Work out the finished part from the listing and answer in its coordinate system (mm). A direction names the side the tool comes from. Coordinates: 2 decimals unless noted, no trailing zeros. Order: outer loops, then holes, each group sorted by start corner. A loop starts at its lowest first (then second) coordinate and runs counter-clockwise, first axis right, second up. Notation, with made-up numbers: (-34, 75.25) -> (-24, 75.25) arc R10 ccw to (-24, 91.25) -> close; hole circle Ø10 at (63.25, -24.75). An arc over 180 degrees is marked (long way). Write item = value, one per line. Start each with the question number.
Q1. The part is cut by section D-D, the plane z = -15. Determine the outline of the cut face in (x, y), plus the area to 3 significant figures.
Q2. Straight lines are drawn through the part: L1, parallel to X at y = -9.75, z = -32.5; L2, parallel to X at y = 1, z = 28.5; L3, parallel to Y at x = 25, z = -16.5. For each, find the intervals that lie inside material, in ascending order. Write a range as from..to.
Q3. Which of the six approach directions +Z, -Z, +X, -X, +Y, -Y give full straight-line access (tool end or side, diameter ignored) to faces 4 (the flat face through (4, -5, 22)), 5 (the cylindrical face through (35.593, -7.168, -40.672)), 6 (the cylindrical face through (4.6, -0.1, 21.8))?
Q4. For a pull along Z with two mould halves and no side action, classify faces 1 (the cylindrical face through (34.73, -7.17, 41.3)), 2 (the flat face through (0, 2, 0)), 3 (the cylindrical face through (15.04, 2.46, -32.63)) as +Z half, -Z half, draft (parallel to the pull), parting line (faces both ways), or undercut.
Q5. Flat-ended cylindrical pins translate along their axes: pin 1 (10 mm diameter, centred on x = 19, y = -16, fed in from -Z); pin 2 (10.5 mm diameter, centred on x = 7, z = 25, fed in from +Y); pin 3 (1.5 mm diameter, centred on x = 33.5, y = 2, fed in from -Z); pin 4 (12 mm diameter, centred on x = 29, z = 32.5, fed in from +Y). Find the tip coordinate at first contact, or state that the pin passes through.
Q6. The part is cut by section A-A, the plane y = -14. Determine the outline of the cut face in (x, z).
Q7. The part is cut by section C-C, the plane x = 29. Determine the outline of the cut face in (y, z), plus the area to 3 significant figures.
Q8. The part is cut by section B-B, the plane x = 7. Determine the outline of the cut face in (y, z).
```python
from build123d import *
from build123d.topology import SkipClean

# Parameters (mm, degrees)
SKETCH1_R                = 4
SKETCH1_R_2              = 7.5
BOSS_EXTRUDE1_DEPTH      = 5
BOSS_EXTRUDE2_START      = -5
SKETCH1_3_R              = 7
SKETCH1_3_R_2            = 4
BOSS_EXTRUDE2_DEPTH      = 5
BOSS_EXTRUDE3_DEPTH      = 5
BOSS_EXTRUDE3_DEPTH_BACK = 19
SKETCH1_4_R              = 10.5
SKETCH1_4_R_2            = 7.5


with BuildPart() as part:
    # Sketch1 → Boss-Extrude1 (new body)
    with BuildSketch(Plane(origin=(0, 0, 0), x_dir=(1, 0, 0), z_dir=(0, 1, 0))):
        with BuildLine():
            Line((2, -30), (2.101020514, -30))
            ThreePointArc((2.101020514, -30), (5.066288205, -31.727611663), (8.496335544, -31.838200051))
            ThreePointArc((8.496335544, -31.838200051), (14.961261821, -32.591823522), (19.59300275, -37.164590308))
            ThreePointArc((19.59300275, -37.164590308), (35.168768008, -40.996840663), (36.348469228, -25))
            ThreePointArc((36.348469228, -25), (25.843366656, 0), (36.348469228, 25))
            ThreePointArc((36.348469228, 25), (35.168768008, 40.996840663), (19.59300275, 37.164590308))
            ThreePointArc((19.59300275, 37.164590308), (14.961261821, 32.591823522), (8.496335544, 31.838200051))
            ThreePointArc((8.496335544, 31.838200051), (2.611056437, 30.45318021), (0, 25))
            Line((0, 25), (0, -25))
            ThreePointArc((0, -25), (0.519259302, -27.645751311), (2, -29.898979486))
            Line((2, -29.898979486), (2, -30))
        make_face()
        with Locations(Location((7, -25, 0), (0, 0, 270))):
            Circle(SKETCH1_R, mode=Mode.SUBTRACT)
        with BuildLine():
            Line((2, 20), (2, 20.101020514))
            ThreePointArc((2, 20.101020514), (2.050252532, 20.050252532), (2.101020514, 20))
            Line((2.101020514, 20), (2, 20))
        make_face(mode=Mode.SUBTRACT)
        with BuildLine():
            ThreePointArc((11.898979486, 20), (11.949747468, 20.050252532), (12, 20.101020514))
            Line((12, 20.101020514), (12, 20))
            Line((12, 20), (11.898979486, 20))
        make_face(mode=Mode.SUBTRACT)
        with Locations(Location((7, 25, 0), (0, 0, 270))):
            Circle(SKETCH1_R, mode=Mode.SUBTRACT)
        with BuildLine():
            ThreePointArc((12, 29.898979486), (11.949747468, 29.949747468), (11.898979486, 30))
            Line((11.898979486, 30), (12, 30))
            Line((12, 30), (12, 29.898979486))
        make_face(mode=Mode.SUBTRACT)
        with Locations(Location((29, 32.5, 0), (0, 0, 270))):
            Circle(SKETCH1_R_2, mode=Mode.SUBTRACT)
        with Locations(Location((29, -32.5, 0), (0, 0, 270))):
            Circle(SKETCH1_R_2, mode=Mode.SUBTRACT)
    extrude(amount=BOSS_EXTRUDE1_DEPTH)

    # Sketch1<3> → Boss-Extrude2 (add)
    # profile 1 of 2: a face of its own
    with BuildSketch(Plane(origin=(0, 0, 0), x_dir=(1, 0, 0), z_dir=(0, 1, 0)).offset(BOSS_EXTRUDE2_START)):
        with Locations(Location((7, 25, 0), (0, 0, 77.657080359))):
            Circle(SKETCH1_3_R)
        with Locations(Location((7, 25, 0), (0, 0, 270))):
            Circle(SKETCH1_3_R_2, mode=Mode.SUBTRACT)
    # profile 2 of 2: a face of its own
    with BuildSketch(Plane(origin=(0, 0, 0), x_dir=(1, 0, 0), z_dir=(0, 1, 0)).offset(BOSS_EXTRUDE2_START)):
        with Locations(Location((7, -25, 0), (0, 0, 180))):
            Circle(SKETCH1_3_R)
        with Locations(Location((7, -25, 0), (0, 0, 270))):
            Circle(SKETCH1_3_R_2, mode=Mode.SUBTRACT)
    extrude(amount=BOSS_EXTRUDE2_DEPTH)

    # Sketch1<4> → Boss-Extrude3 (add, two sides: drawn at the far end of the back side and taken through both)
    # profile 1 of 2: a face of its own
    with SkipClean():  # the faces are left unmerged after this step: merging them gives an invalid solid
        with BuildSketch(Plane(origin=(0, 0, 0), x_dir=(1, 0, 0), z_dir=(0, 1, 0)).offset(-BOSS_EXTRUDE3_DEPTH_BACK)):
            with Locations(Location((29, 32.5, 0), (0, 0, 153.62484734))):
                Circle(SKETCH1_4_R)
            with Locations(Location((29, 32.5, 0), (0, 0, 270))):
                Circle(SKETCH1_4_R_2, mode=Mode.SUBTRACT)
        # profile 2 of 2: a face of its own
        with BuildSketch(Plane(origin=(0, 0, 0), x_dir=(1, 0, 0), z_dir=(0, 1, 0)).offset(-BOSS_EXTRUDE3_DEPTH_BACK)):
            with Locations(Location((29, -32.5, 0), (0, 0, 45.584691403))):
                Circle(SKETCH1_4_R)
            with Locations(Location((29, -32.5, 0), (0, 0, 270))):
                Circle(SKETCH1_4_R_2, mode=Mode.SUBTRACT)
        extrude(amount=BOSS_EXTRUDE3_DEPTH + BOSS_EXTRUDE3_DEPTH_BACK)


solid = part.part
```
Model answer:
q1.outline = (0, 0) -> (29.22, 0) -> (29.22, 5) -> (0, 5) -> close
q1.area = 146 mm2
q2.L1 = 18.5..21.5, 36.5..39.5
q2.L2 = 0.94..5.06, 8.94..22.66, 35.34..38.71
q2.L3 = 0..5
q3.face_4 = +Z, -Z, -X, -Y
q3.face_5 = -Y
q3.face_6 = +Y, -Y
q4.face_1 = undercut
q4.face_2 = draft
q4.face_3 = -Z half
q5.pin_1 = -41.73
q5.pin_2 = 5
q5.pin_3 = -42.31
q5.pin_4 = through
q6.outline = circle Ø21 at (29, -32.5); circle Ø21 at (29, 32.5); hole circle Ø15 at (29, -32.5); hole circle Ø15 at (29, 32.5)
q7.outline = (-19, -43) -> (5, -43) -> (5, -40) -> (-19, -40) -> close; (-19, -25) -> (5, -25) -> (5, -14.53) -> (0, -14.53) -> (0, -22) -> (-19, -22) -> close; (-19, 22) -> (0, 22) -> (0, 14.53) -> (5, 14.53) -> (5, 25) -> (-19, 25) -> close; (-19, 40) -> (5, 40) -> (5, 43) -> (-19, 43) -> close
q7.area = 363 mm2
q8.outline = (-5, -32) -> (5, -32) -> (5, -29) -> (-5, -29) -> close; (-5, -21) -> (5, -21) -> (5, 21) -> (-5, 21) -> (-5, 18) -> (0, 18) -> (0, -18) -> (-5, -18) -> close; (-5, 29) -> (5, 29) -> (5, 32) -> (-5, 32) -> close
